Geometry: see drawing. Coordinates: mm, zero at the bounding-box minimum. Round coordinates to 2 decimals unless told otherwise and drop trailing zeros. Loops run counter-clockwise (first coordinate to the right, second up) from the corner with the lowest first, then second, coordinate; pieces in that order, holes last.
(1) Draft query along Y for the marked faces 1, 2 and 3. Return one class per face: released by +Y, released by -Y, zero draft, split by the parting line, or undercut.
(2) Line query: line 1 (X direction, y = 10.25, z = 2.75); line 2 (Y direction, x = 0.75, z = 4.6); line 3 (X direction, y = 10.5, z = 2.75). Output: solid intervals per line, ascending.
(3) Cut plane A-A, the plane z = 0.95. Output: boundary loops of the cut face in (x, y).
(4) Cut plane B-B, the plane y = 10.5. Output: boundary loops of the cut face in (x, z), and give its area (4 significant figures).
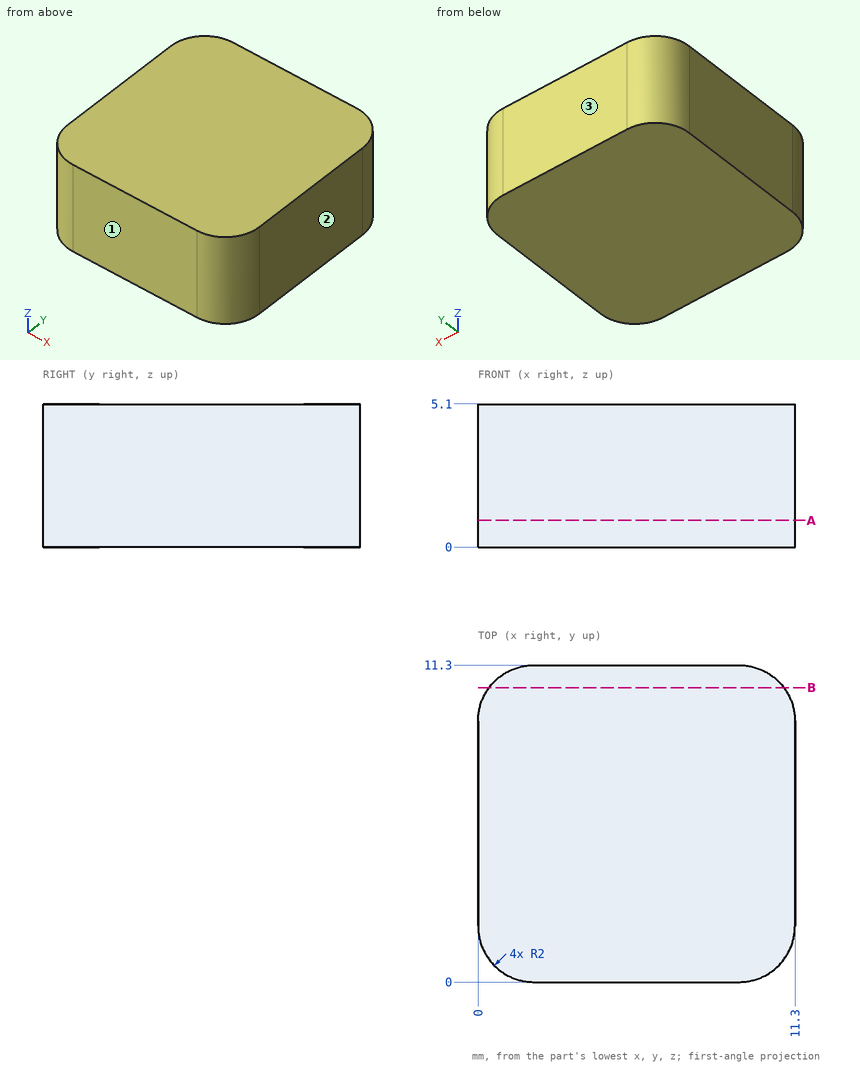
Reported:
1. face 1: released by -Y
1. face 2: zero draft
1. face 3: released by +Y
2. line 1: x = 0.24 to 11.06
2. line 2: y = 0.44 to 10.86
2. line 3: x = 0.4 to 10.9
3. outline: (0, 2) arc R2 ccw to (2, 0) - (9.3, 0) arc R2 ccw to (11.3, 2) - (11.3, 9.3) arc R2 ccw to (9.3, 11.3) - (2, 11.3) arc R2 ccw to (0, 9.3) - close
4. outline: (0.4, 0) - (10.9, 0) - (10.9, 5.1) - (0.4, 5.1) - close
4. area: 53.55 mm2
